Part model, mm, in its own coordinate system. A direction names the side the tool comes from. Give positions to 0.01 mm unless a question says otherwise; leave off trailing zeros. Order: outer loops, then holes, each group sorted by start corner. A loop starts at its lowest first (then second) coordinate and runs counter-clockwise, first axis right, second up. Notation, with made-up numbers: M -13,38 L 15,38 A15 ccw 15,42 Z; hole C -21.5,79.5 d6. An arc over 180 degrees is marked long. Return JSON: item names as keys, results as strings.
from build123d import *

# Parameters (mm, degrees)
SKETCH1_R             = 1.905
BOSS_EXTRUDE1_DEPTH   = 4.445
BOSS_EXTRUDE1_2_DEPTH = 4.445
BOSS_EXTRUDE1_3_DEPTH = 4.445
SKETCH1_R_2           = 1.27
BOSS_EXTRUDE1_4_DEPTH = 4.445
SKETCH2_W             = 6.731
SKETCH2_H             = 13.97
BOSS_EXTRUDE2_DEPTH   = 12.7
CHAMFER1_SIZE         = 3.81
SKETCH3_R             = 5.3975
BOSS_EXTRUDE3_DEPTH   = 3.429
SKETCH4_R             = 4.7625
BOSS_EXTRUDE4_DEPTH   = 13.843
FILLET1_R             = 2.54
FILLET2_R             = 1.27


with BuildPart() as part:
    # Sketch1 → Boss-Extrude1 (new body)
    with BuildSketch(Plane(origin=(0, 0, 0), x_dir=(1, 0, 0), z_dir=(0, 1, 0))):
        with Locations((0.635, 5.08)):
            Circle(SKETCH1_R)
    extrude(amount=-BOSS_EXTRUDE1_DEPTH)



with BuildPart() as body_2:
    # Sketch1 → Boss-Extrude1 2 (new body)
    with BuildSketch(Plane(origin=(0, 0, 0), x_dir=(1, 0, 0), z_dir=(0, 1, 0))):
        with Locations((0.635, -5.08)):
            Circle(SKETCH1_R)
    extrude(amount=-BOSS_EXTRUDE1_2_DEPTH)


with BuildPart() as body_3:
    # Sketch1 → Boss-Extrude1 3 (new body)
    with BuildSketch(Plane(origin=(0, 0, 0), x_dir=(1, 0, 0), z_dir=(0, 1, 0))):
        with Locations((5.715, 0)):
            Circle(SKETCH1_R)
    extrude(amount=-BOSS_EXTRUDE1_3_DEPTH)


with BuildPart() as body_4:
    # Sketch1 → Boss-Extrude1 4 (new body)
    with BuildSketch(Plane(origin=(0, 0, 0), x_dir=(1, 0, 0), z_dir=(0, 1, 0))):
        Circle(SKETCH1_R_2)
    extrude(amount=-BOSS_EXTRUDE1_4_DEPTH)


with BuildPart() as part_1:
    add(part.part)

    add(body_2.part)  # Boss-Extrude2 merges body 2

    add(body_3.part)  # Boss-Extrude2 merges body 3

    add(body_4.part)  # Boss-Extrude2 merges body 4
    # Sketch2 → Boss-Extrude2 (add)
    with BuildSketch(Plane(origin=(0, 0, 0), x_dir=(-1, 0, 0), z_dir=(0, 1, 0))):
        with Locations((-2.3495, 0)):
            Rectangle(SKETCH2_W, SKETCH2_H)
    extrude(amount=BOSS_EXTRUDE2_DEPTH)

    # Chamfer1
    chamfer1_edges = [part_1.edges().sort_by_distance(p)[0] for p in [
        (-1.016, 12.7, 0),
    ]]
    chamfer(chamfer1_edges, length=CHAMFER1_SIZE)

    # Sketch3 → Boss-Extrude3 (add)
    with BuildSketch(Plane(origin=(5.715, 0, 0), x_dir=(0, 0, -1), z_dir=(1, 0, 0))):
        with Locations((0, 7.0485)):
            Circle(SKETCH3_R)
    extrude(amount=BOSS_EXTRUDE3_DEPTH)

    # Sketch4 → Boss-Extrude4 (add)
    with BuildSketch(Plane(origin=(9.144, 0, 0), x_dir=(0, 0, -1), z_dir=(1, 0, 0))):
        with Locations((0, 7.0485)):
            Circle(SKETCH4_R)
    extrude(amount=BOSS_EXTRUDE4_DEPTH)

    # Fillet1
    fillet1_edges = [part_1.edges().sort_by_distance(p)[0] for p in [
        (22.987, 7.0485, 4.7625),
    ]]
    fillet(fillet1_edges, radius=FILLET1_R)

    # Fillet2
    fillet2_edges = [part_1.edges().sort_by_distance(p)[0] for p in [
        (-1.27, -4.445, 5.08),
        (3.81, -4.445, 0),
        (-1.27, -4.445, 0),
        (-1.27, -4.445, -5.08),
    ]]
    fillet(fillet2_edges, radius=FILLET2_R)


solid = part_1.part
Q1. Band-saw the part on A-A (x = 13). Give the cut face in (y, z) (1 decimal), then the cut area to 3 significant figures.
Established:
{"outline": "C 7,0 d9.5", "area": "71.3 mm²"}
Q2. Two-plate mould, pull along X, no slides. Class faces 5 (the flat face through (22.987, 7, 0)), 6 (the cylindrical face through (-0.17, -1.57, -1.26)), 7 (the flat face through (-0.61, 0, -6.72)): +X half, -X half, draft (parallel to the pull), parting line (faces both ways), or undercut.
Established:
{"face 5": "+X half", "face 6": "undercut", "face 7": "draft"}
Q3. Pin check, flat tips, straight feed: pin 1 (1.5 mm diameter, centred on x = 7, z = -1, fed in from +Y); pin 2 (8 mm diameter, centred on x = 13, y = -1, fed in from +Z); pin 3 (1 mm diameter, centred on y = 5.5, z = 3.5, fed in from +X). Stop position of each tip, or through.
Established:
{"pin 1": "stops at y = 12.44", "pin 2": "stops at z = 2.51", "pin 3": "stops at x = 22.73"}
Q4. Probe line 1 along X through (y, z) = (5.5, -4.75); line 2 along X through (y, z) = (-3.5, -0.75); line 3 along Y through (x, z) = (7.5, 0). List the from-to ranges inside material, lowest first.
Established:
{"line 1": "x = -1.02 to 9.14", "line 2": "x = -0.97 to 0.97, 4.01 to 7.42", "line 3": "y = -3.71 to 0, 1.65 to 12.45"}
Q5. 3-axis set-ups, long thin cutter, end or side, ignore diameter. For faces 1 (the flat face through (-0.61, 0, 6.72)), 2 (the cylindrical face through (3.81, -1.57, -0.08)), 3 (the flat face through (-1.016, 4, 0)), 4 (the flat face through (9.144, 2, 0)): which of +Z, -Z, +X, -X, +Y, -Y reach the whole face in a straight line?
Established:
{"face 1": "+Z, -X, -Y", "face 2": "-Y", "face 3": "+Z, -Z, -X, +Y", "face 4": "+X"}
